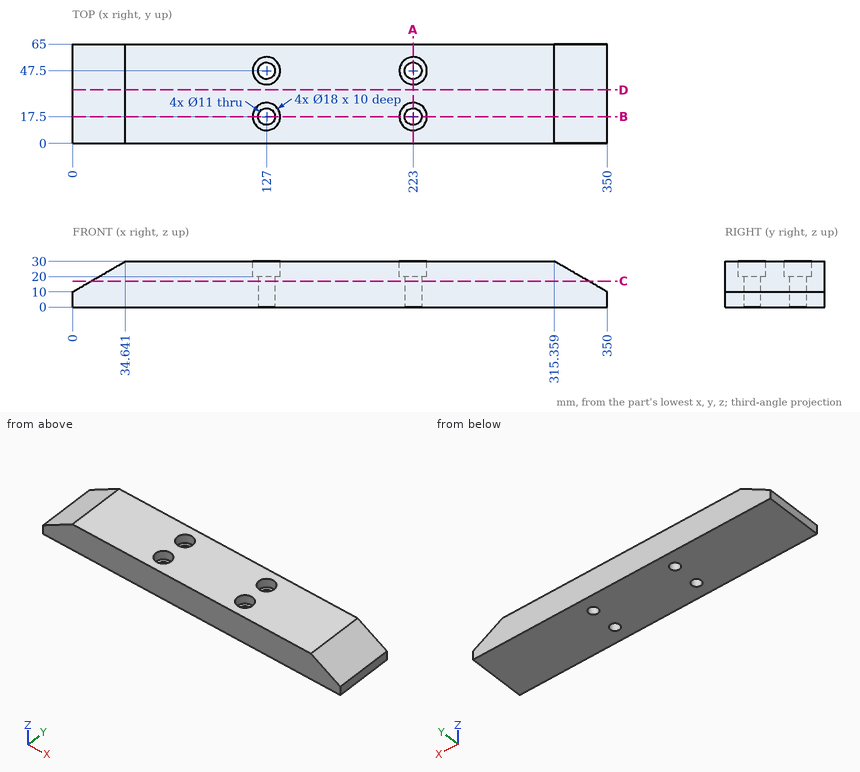
Can you work these out from the drawing? Everything is in mm from the part's minimum corner. Round coordinates to 2 decimals unless told otherwise and drop trailing zeros. Order: outer loops, then holes, each group sorted by start corner. A loop starts at its lowest first (then second) coordinate and runs counter-clockwise, first axis right, second up.
(1) If we section it at B-B (y = 17.5): Please give me the cut outline in (x, z), plus the area to 3 significant figures.
Results are:
outline: (0, 0) - (121.5, 0) - (121.5, 20) - (118, 20) - (118, 30) - (34.64, 30) - (0, 10) - close; (132.5, 0) - (217.5, 0) - (217.5, 20) - (214, 20) - (214, 30) - (136, 30) - (136, 20) - (132.5, 20) - close; (228.5, 0) - (350, 0) - (350, 10) - (315.36, 30) - (232, 30) - (232, 20) - (228.5, 20) - close
area: 9,010 mm2
(2) I'm going to push flat-ended pins straight in: pin 1 (5.5 mm diameter, centred on x = 127.5, y = 46, fed in from +Z); pin 2 (16 mm diameter, centred on x = 127, y = 47.5, fed in from +Z); pin 3 (6 mm diameter, centred on y = 11, z = 21, fed in from +X); pin 4 (1 mm diameter, centred on y = 38.5, z = 12.5, fed in from +X). Where does each tip first touch, or does it pass through?
Results are:
pin 1: passes through
pin 2: stops at z = 20
pin 3: stops at x = 336.14
pin 4: stops at x = 346.54
(3) If we section it at D-D (y = 35): Please give me the cut outline in (x, z).
Results are:
outline: (0, 0) - (350, 0) - (350, 10) - (315.36, 30) - (34.64, 30) - (0, 10) - close
(4) If we section it at C-C (z = 17): Please give me the cut outline in (x, y).
Results are:
outline: (12.12, 0) - (337.88, 0) - (337.88, 65) - (12.12, 65) - close; hole circle Ø11 at (127, 17.5); hole circle Ø11 at (127, 47.5); hole circle Ø11 at (223, 17.5); hole circle Ø11 at (223, 47.5)
(5) If I drill on L1, parallel to Y at x = 127, z = 23; L2, parallel to Y at x = 127, z = 12.5; L3, parallel to X at y = 17, z = 23, over which ranges is the centre line in solid material (lowest first)?
Results are:
L1: y = 0 to 8.5, 26.5 to 38.5, 56.5 to 65
L2: y = 0 to 12, 23 to 42, 53 to 65
L3: x = 22.52 to 118.01, 135.99 to 214.01, 231.99 to 327.48
(6) If we section it at A-A (x = 223): Please give me the cut outline in (y, z).
Results are:
outline: (0, 0) - (12, 0) - (12, 20) - (8.5, 20) - (8.5, 30) - (0, 30) - close; (23, 0) - (42, 0) - (42, 20) - (38.5, 20) - (38.5, 30) - (26.5, 30) - (26.5, 20) - (23, 20) - close; (53, 0) - (65, 0) - (65, 30) - (56.5, 30) - (56.5, 20) - (53, 20) - close
